Here's the drawing with two shaded views (mm, measured from the low corner). I have some questions. A direction names the side the tool comes from. Give positions to 0.01 mm unless a question says otherwise; leave off trailing zeros. Write each loop counter-clockwise with the first axis right and the second up, starting at its lowest first coordinate (ties: lowest second). Pieces come first, ordered by that corner, then holes.
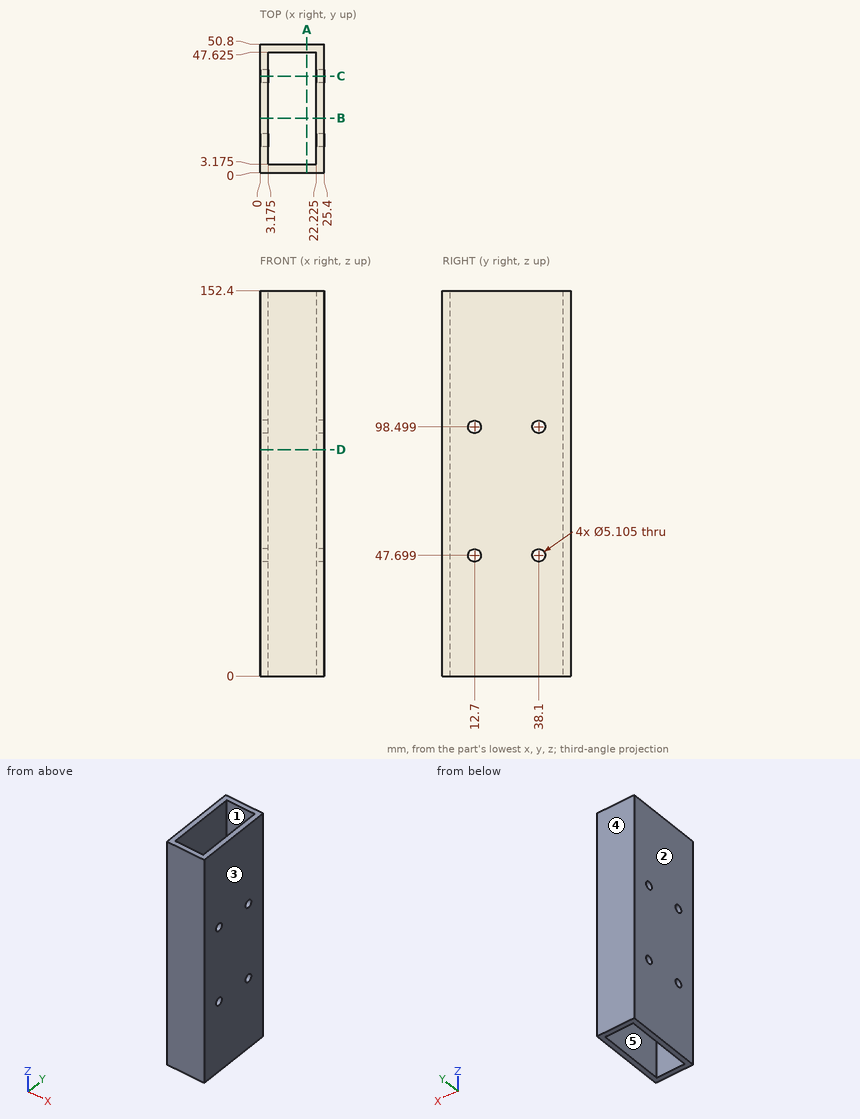
(1) If we mould it in two halves opening along Y, with no side actions, what happens to the marked faces 3, 4 and 5? For each: +Y half, -Y half, draft (parallel to the pull), parting line (faces both ways), or undercut.
Returned:
face 3: draft
face 4: +Y half
face 5: undercut
(2) Imagine slicing it at D-D, the plane z = 89.5. Write out the boundary of the cut face in (x, y) (1 decimal).
Returned:
outline: (0, 0) - (25.4, 0) - (25.4, 50.8) - (0, 50.8) - close; hole (3.2, 3.2) - (22.2, 3.2) - (22.2, 47.6) - (3.2, 47.6) - close
(3) Imagine slicing it at C-C, the plane y = 38.1. Write out the boundary of the cut face in (x, z) (1 decimal).
Returned:
outline: (0, 0) - (3.2, 0) - (3.2, 45.1) - (0, 45.1) - close; (0, 50.3) - (3.2, 50.3) - (3.2, 95.9) - (0, 95.9) - close; (0, 101.1) - (3.2, 101.1) - (3.2, 152.4) - (0, 152.4) - close; (22.2, 0) - (25.4, 0) - (25.4, 45.1) - (22.2, 45.1) - close; (22.2, 50.3) - (25.4, 50.3) - (25.4, 95.9) - (22.2, 95.9) - close; (22.2, 101.1) - (25.4, 101.1) - (25.4, 152.4) - (22.2, 152.4) - close
(4) If I drill on L1, parallel to Z at x = 24.15, y = 38.1; L2, parallel to X at y = 44, z = 36.5 (1 decimal); L3, parallel to Y at x = 19.25, z = 72 (1 decimal), over which ranges is the centre line in solid material (lowest first)?
Returned:
L1: z = 0 to 45.15, 50.25 to 95.95, 101.05 to 152.4
L2: x = 0 to 3.2, 22.2 to 25.4
L3: y = 0 to 3.2, 47.6 to 50.8
(5) Imagine slicing it at B-B, the plane y = 21.5. Write out the boundary of the cut face in (x, z) (1 decimal).
Returned:
outline: (0, 0) - (3.2, 0) - (3.2, 152.4) - (0, 152.4) - close; (22.2, 0) - (25.4, 0) - (25.4, 152.4) - (22.2, 152.4) - close
(6) Imagine slicing it at A-A, the plane x = 18.5. Write out the boundary of the cut face in (y, z) (1 decimal).
Returned:
outline: (0, 0) - (3.2, 0) - (3.2, 152.4) - (0, 152.4) - close; (47.6, 0) - (50.8, 0) - (50.8, 152.4) - (47.6, 152.4) - close
(7) For the marked faces 1 and 2, which set-ups out of +Z, -Z, +X, -X, +Y, -Y let a thin tool reach every point of the face, with its end or its side?
Returned:
face 1: +Z, -Z
face 2: +Z, -Z, -X, +Y, -Y
